Verification items for the finished model (mm, model axes). A direction names the side the tool comes from. Coordinates: 2 decimals unless noted, no trailing zeros. Order: outer loops, then holes, each group sorted by start corner. A loop starts at its lowest first (then second) coordinate and runs counter-clockwise, first axis right, second up. Notation, with made-up numbers: M 7.25,-12.75 L 59.25,-12.75 A24 cw 59.25,12.25 Z; hole C 19.25,-12 d10. An arc over 180 degrees is marked long. Answer as a JSON object with one key per item and string values. Group by question number.
(1) Cross-section at B-B (y = 80). Enter the section's corners in (x, z), plus the area to 3 significant figures.
(2) Cross-section at A-A (z = 13). Enter the section's corners in (x, y), plus the area to 3 significant figures.
(3) Mould release check, pull along Y, two halves, no side actions. Record for faces 3 (the face through (-32, 35, 0)), 4 (the face through (27.94, 165, 12.52)), 5 (the face through (-142.594, -4.046, 12.522)): released by +Y, released by -Y, zero draft, split by the parting line, or undercut.
(4) Cross-section at D-D (x = 56.5). Enter the section's corners in (y, z).
(5) Access from +Z, -Z, +X, -X, +Y, -Y to the whole of each face (thin tool, end or side, straight path). Record for faces 1 (the face through (150, 20.238, 13)), 2 (the face through (174.295, -1.348, 12.522)).
(6) Gauge pin test, flat ends, axial feed: pin 1 Ø15 at (x, y) = (85.98, 71.04) entering from +Z; pin 2 Ø1.5 at (y, z) = (147.5, 13) entering from -X; pin 3 Ø7.5 at (y, z) = (139.5, 9.5) entering from +X; pin 4 Ø10 at (x, z) = (148.5, 17.5) entering from +Y. Record the tip position at first contact, or that the pin passes through.
(7) Cross-section at C-C (y = -10). Enter the section's corners in (x, z), plus the area to 3 significant figures.
(8) Material ranges on line 1 (Y direction, x = -121.5, z = 23.25); line 2 (Y direction, x = -99, z = 23.25); line 3 (Y direction, x = 68, z = 12), recorded low to high.
from build123d import *

# Parameters (mm, degrees)
F0_R     = 25.4
F0_R_2   = 12.7
F1_DEPTH = 25.4


with BuildPart() as f1:
    # F0 (on Top) → F1 (new body)
    with BuildSketch(Plane.XY):
        with BuildLine():
            Line((-117.218833, -55.96244), (162.181167, -55.96244))
            ThreePointArc((162.181167, -55.96244), (180.141679, -48.522952), (187.581167, -30.56244))
            Line((187.581167, -30.56244), (187.581167, -5.16244))
            ThreePointArc((187.581167, -5.16244), (180.141679, 12.798073), (162.181167, 20.23756))
            Line((162.181167, 20.23756), (136.781167, 20.23756))
            ThreePointArc((136.781167, 20.23756), (118.820655, 27.677048), (111.381167, 45.63756))
            Line((111.381167, 45.63756), (111.381167, 71.03756))
            ThreePointArc((111.381167, 71.03756), (103.941679, 88.998073), (85.981167, 96.43756))
            Line((85.981167, 96.43756), (60.581167, 96.43756))
            ThreePointArc((60.581167, 96.43756), (42.620655, 103.877048), (35.181167, 121.83756))
            Line((35.181167, 121.83756), (35.181167, 147.23756))
            ThreePointArc((35.181167, 147.23756), (27.741679, 165.198073), (9.781167, 172.63756))
            Line((9.781167, 172.63756), (-117.218833, 172.63756))
            ThreePointArc((-117.218833, 172.63756), (-153.139857, 157.758585), (-168.018833, 121.83756))
            Line((-168.018833, 121.83756), (-168.018833, -5.16244))
            ThreePointArc((-168.018833, -5.16244), (-153.139857, -41.083464), (-117.218833, -55.96244))
        make_face()
        with Locations((-117.218833, -5.16244)):
            Circle(F0_R, mode=Mode.SUBTRACT)
        with Locations((162.181167, -5.16244)):
            Circle(F0_R_2, mode=Mode.SUBTRACT)
        with Locations((-117.218833, 121.83756)):
            Circle(F0_R, mode=Mode.SUBTRACT)
        with Locations((9.781167, 147.23756)):
            Circle(F0_R_2, mode=Mode.SUBTRACT)
        with Locations((85.981167, 71.03756)):
            Circle(F0_R_2, mode=Mode.SUBTRACT)
    extrude(amount=F1_DEPTH)


solid = f1.part
Taken from the geometry:
{
 "1": {"outline": "M -168.02,0 L 76.98,0 L 76.98,25.4 L -168.02,25.4 Z; M 94.98,0 L 109.75,0 L 109.75,25.4 L 94.98,25.4 Z", "area": "6,600 mm²"},
 "2": {"outline": "M -168.02,-5.16 A50.8 ccw -117.22,-55.96 L 162.18,-55.96 A25.4 ccw 187.58,-30.56 L 187.58,-5.16 A25.4 ccw 162.18,20.24 L 136.78,20.24 A25.4 cw 111.38,45.64 L 111.38,71.04 A25.4 ccw 85.98,96.44 L 60.58,96.44 A25.4 cw 35.18,121.84 L 35.18,147.24 A25.4 ccw 9.78,172.64 L -117.22,172.64 A50.8 ccw -168.02,121.84 Z; hole C -117.22,-5.16 d50.8; hole C -117.22,121.84 d50.8; hole C 9.78,147.24 d25.4; hole C 85.98,71.04 d25.4; hole C 162.18,-5.16 d25.4", "area": "56,900 mm²"},
 "3": {"face 3": "zero draft", "face 4": "released by +Y", "face 5": "undercut"},
 "4": {"outline": "M -55.96,0 L 96.77,0 L 96.77,25.4 L -55.96,25.4 Z"},
 "5": {"face 1": "+Z, -Z, +X, +Y", "face 2": "+Z, -Z"},
 "6": {"pin 1": "passes through", "pin 2": "stops at x = -161.49", "pin 3": "stops at x = 35.18", "pin 4": "stops at y = 20.24"},
 "7": {"outline": "M -167.79,0 L -142.15,0 L -142.15,25.4 L -167.79,25.4 Z; M -92.28,0 L 150.44,0 L 150.44,25.4 L -92.28,25.4 Z; M 173.92,0 L 187.58,0 L 187.58,25.4 L 173.92,25.4 Z", "area": "7,160 mm²"},
 "8": {"line 1": "y = -55.78 to -30.2, 19.87 to 96.8, 146.87 to 172.46", "line 2": "y = -55.96 to -22.86, 12.54 to 104.14, 139.54 to 172.64", "line 3": "y = -55.96 to 96.44"}
}
